Job drawing, mm, ordinate dimensions from the low corner. One solid piece. Round coordinates to 2 decimals unless told otherwise and drop trailing zeros. Order: outer loops, then holes, each group sorted by start corner. A loop starts at its lowest first (then second) coordinate and runs counter-clockwise, first axis right, second up. Notation, with made-up numbers: M 71.5,39 L 120.5,39 A6 ccw 120.5,46 Z; hole C -17.5,83.5 d1. An arc over 180 degrees is marked long. Answer as a JSON object with one key per item and string values. Group by question number.
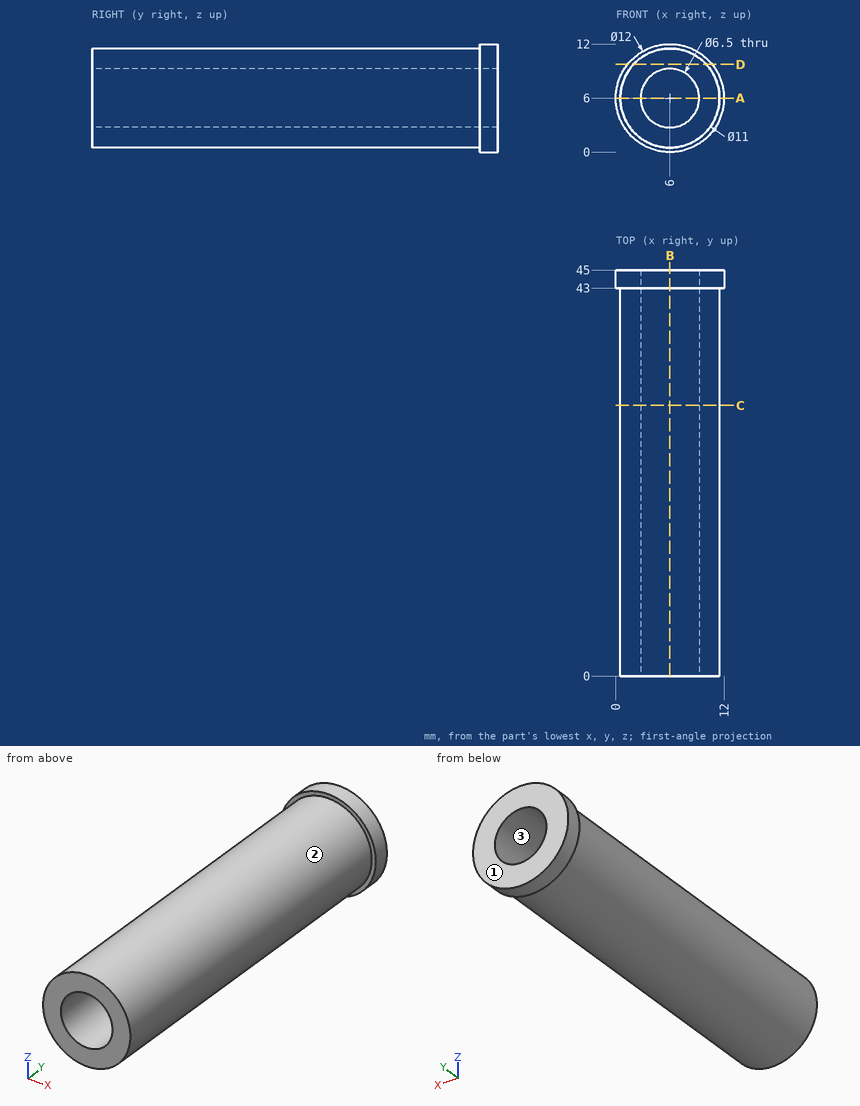
Item 1: Cut at A-A, the plane z = 6. Give the cut face in (x, y), and give its area (4 significant figures).
Item 2: Drill centre lines: line 1 (X direction, y = 19.5, z = 6); line 2 (X direction, y = 10, z = 7.25). Where is each one in solid material? Low to high. Write a range as [from, to].
Item 3: Cut at C-C, the plane y = 30. Give the cut face in (x, z).
Item 4: Cut at D-D, the plane z = 9.75. Give the cut face in (x, y).
Item 5: Flat gauge pins, fed straight in: pin 1 Ø1.5 at (x, y) = (6, 10.5) entering from -Z; pin 2 Ø2 at (x, y) = (9.5, 14) entering from +Z; pin 3 Ø2 at (y, z) = (21, 8) entering from +X. Where does each tip first touch, or does it go through?
Item 6: Cut at B-B, the plane x = 6. Give the cut face in (y, z).
Item 7: Two-plate mould, pull along Z, no slides. Class the marked faces 1, 2 and 3: +Z half, -Z half, draft (parallel to the pull), parting line (faces both ways), or undercut.
Response values:
{
 "1": {"outline": "M 0,43 L 0.5,43 L 0.5,0 L 2.75,0 L 2.75,45 L 0,45 Z; M 9.25,0 L 11.5,0 L 11.5,43 L 12,43 L 12,45 L 9.25,45 Z", "area": "204.5 mm^2"},
 "2": {"line 1": "[0.5, 2.75], [9.25, 11.5]", "line 2": "[0.64, 3], [9, 11.36]"},
 "3": {"outline": "C 6,6 d11; hole C 6,6 d6.5"},
 "4": {"outline": "M 1.32,43 L 1.98,43 L 1.98,0 L 10.02,0 L 10.02,43 L 10.68,43 L 10.68,45 L 1.32,45 Z"},
 "5": {"pin 1": "z = 0.5", "pin 2": "z = 10.9", "pin 3": "x = 11.41"},
 "6": {"outline": "M 0,0.5 L 43,0.5 L 43,0 L 45,0 L 45,2.75 L 0,2.75 Z; M 0,9.25 L 45,9.25 L 45,12 L 43,12 L 43,11.5 L 0,11.5 Z"},
 "7": {"face 1": "draft", "face 2": "parting line", "face 3": "undercut"}
}
